Here's how the part is built. I have some questions about the finished solid (model axes, mm). Round coordinates to 2 decimals unless told otherwise and drop trailing zeros. Loops run counter-clockwise (first coordinate to the right, second up) from the corner with the lowest first, then second, coordinate; pieces in that order, holes last. Notation, with made-up numbers: (44.5, 68.25) - (59.5, 68.25) arc R35 ccw to (59.5, 105.25) - close; hole circle Ø2 at (-14, 13.25). An arc over 180 degrees is marked (long way). Answer as a JSON object with one key per item and string values. Group by question number.
1) I want a section at A-A, the plane x = 195.58. Please give me the cut outline in (y, z), then the cut area to 3 significant figures.
2) I want a section at C-C, the plane z = 0.65. Give the number of separate pieces and of enclosed holes in the cut face, then the cut area to 3 significant figures.
3) I want a section at B-B, the plane y = 112. Please give me the cut outline in (x, z).
4) If I drill on line 1 along Y through (x, z) = (110.49, 3.2); line 2 along Y through (x, z) = (214.99, 3.1); line 3 along Y through (x, z) = (204.47, 1.65), over which ranges is the centre line in solid material (lowest first)? Write a range as [from, to].
from build123d import *

# Parameters (mm, degrees)
F0_W     = 220.98
F0_H     = 220.98
F1_DEPTH = 4.2672
F3_D     = 2.2606
F5_DEPTH = 4.2682
F7_D     = 3.4
F9_D     = 3.4


with BuildPart() as f1:
    # F0 (on Top) → F1 (new body)
    with BuildSketch(Plane.XY):
        with Locations((110.49, 110.49)):
            Rectangle(F0_W, F0_H)
    extrude(amount=F1_DEPTH)

    # F3 (through all)
    with Locations(Plane.XY.offset(4.2672)):
        with Locations((5.99, 214.99), (214.99, 214.99), (214.99, 5.99), (5.99, 5.99)):
            Hole(F3_D / 2)

    # F4 (on face) → F5 (cut, through all)
    with BuildSketch(Plane.XY.offset(4.2672)):
        with BuildLine():
            ThreePointArc((30.1625, 122.555), (25.4, 127.3175), (20.6375, 122.555))
            Line((20.6375, 122.555), (20.6375, 98.425))
            ThreePointArc((20.6375, 98.425), (25.4, 93.6625), (30.1625, 98.425))
            Line((30.1625, 98.425), (30.1625, 122.555))
        make_face()
        with BuildLine():
            ThreePointArc((200.3425, 78.105), (195.58, 82.8675), (190.8175, 78.105))
            Line((190.8175, 78.105), (190.8175, 53.975))
            ThreePointArc((190.8175, 53.975), (195.58, 49.2125), (200.3425, 53.975))
            Line((200.3425, 53.975), (200.3425, 78.105))
        make_face()
        with BuildLine():
            Line((200.3425, 142.875), (200.3425, 167.005))
            ThreePointArc((200.3425, 167.005), (195.58, 171.7675), (190.8175, 167.005))
            Line((190.8175, 167.005), (190.8175, 142.875))
            ThreePointArc((190.8175, 142.875), (195.58, 138.1125), (200.3425, 142.875))
        make_face()
    extrude(amount=-F5_DEPTH, mode=Mode.SUBTRACT)

    # F7 (through all)
    with Locations(Plane.XY.offset(4.2672)):
        with Locations((110.49, 130.99), (110.49, 89.99)):
            Hole(F7_D / 2)

    # F9 (through all)
    with Locations(Plane.XY.offset(4.2672)):
        with Locations((16.51, 118.4275), (16.51, 102.5525), (34.29, 118.4275), (34.29, 102.5525), (204.47, 162.8775), (186.69, 147.0025), (186.69, 162.8775), (204.47, 147.0025), (204.47, 73.9775), (186.69, 58.1025), (204.47, 58.1025), (186.69, 73.9775)):
            Hole(F9_D / 2)


solid = f1.part
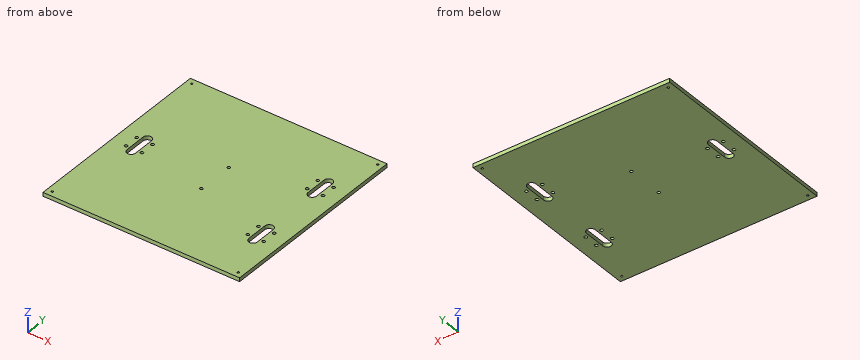
Outcome:
{
 "1": {"outline": "(0, 0) - (49.21, 0) - (49.21, 4.27) - (0, 4.27) - close; (82.87, 0) - (138.11, 0) - (138.11, 4.27) - (82.87, 4.27) - close; (171.77, 0) - (220.98, 0) - (220.98, 4.27) - (171.77, 4.27) - close", "area": "656 mm^2"},
 "2": {"separate pieces": "1", "enclosed holes": "21", "area": "47,800 mm^2"},
 "3": {"outline": "(0, 0) - (20.64, 0) - (20.64, 4.27) - (0, 4.27) - close; (30.16, 0) - (220.98, 0) - (220.98, 4.27) - (30.16, 4.27) - close"},
 "4": {"line 1": "[0, 88.29], [91.69, 129.29], [132.69, 220.98]", "line 2": "[0, 4.86], [7.12, 213.86], [216.12, 220.98]", "line 3": "[0, 56.4], [59.8, 72.28], [75.68, 145.3], [148.7, 161.18], [164.58, 220.98]"}
}
